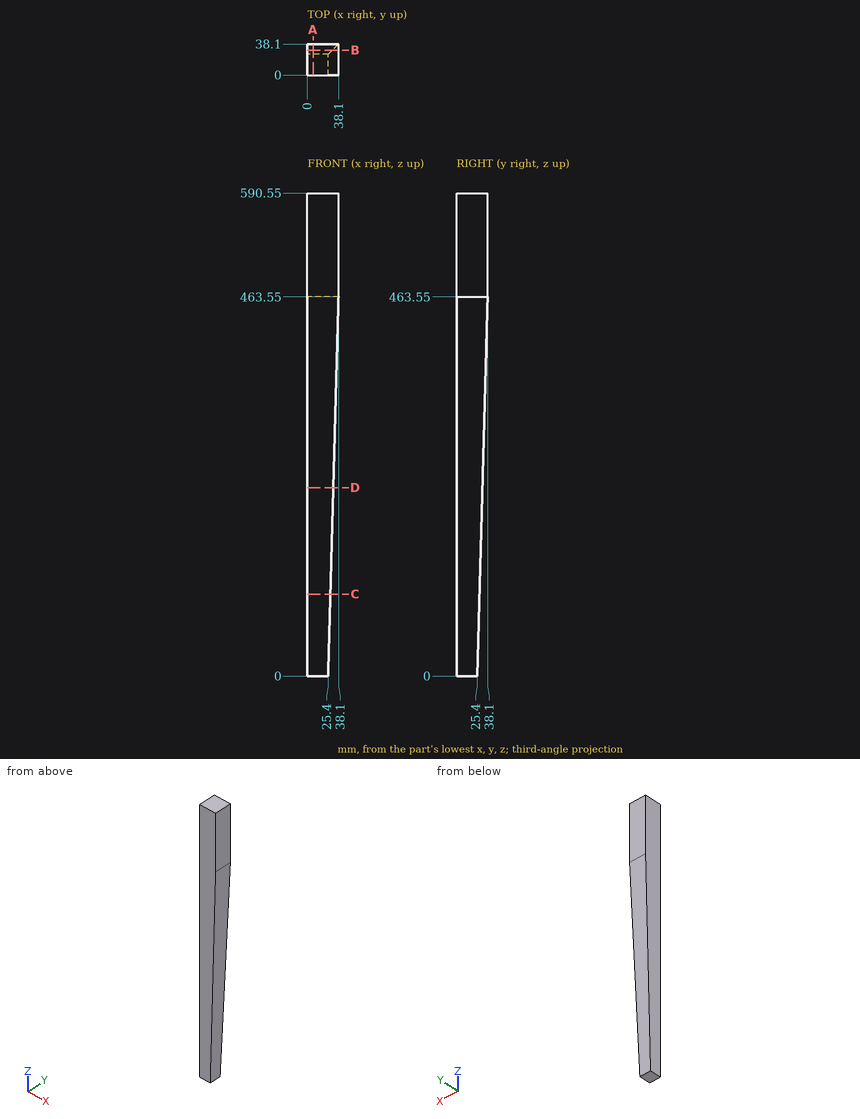
Source: three-view drawing plus pictorial views. Frame: mm from the lowest corner of the part. Round coordinates to 2 decimals unless told otherwise and drop trailing zeros. Order: outer loops, then holes, each group sorted by start corner. A loop starts at its lowest first (then second) coordinate and runs counter-clockwise, first axis right, second up. Notation, with made-up numbers: (7.5, 18.25) -> (33.5, 18.25) arc R24 ccw to (33.5, 57.25) -> close; hole circle Ø10 at (-16, 69). An arc over 180 degrees is marked (long way). Use one line per item in the form item = value. Start each with the question number.
1. Cut plane A-A (x = 7). Return the cut outline in (y, z), then the cut area to 3 significant figures.
2. Pin query (flat end, axial travel): pin 1 Ø4 at (x, z) = (23, 325.5) entering from +Y. Return the tip coordinate at first contact, or that it passes through.
3. Line query: probe 1 along X at (y, z) = (10, 186); probe 2 along X at (y, z) = (2, 153.5); probe 3 along Y at (x, z) = (21.5, 189). Output: solid intervals per line, ascending.
4. Cut plane B-B (y = 30.5). Return the cut outline in (x, z), then the cut area to 3 significant figures.
5. Cut plane C-C (z = 100). Return the cut outline in (x, y), then the cut area to 3 significant figures.
6. Cut plane D-D (z = 230.5). Return the cut outline in (x, y), then the cut area to 3 significant figures.
Solution:
q1.outline = (0, 0) -> (25.4, 0) -> (38.1, 463.55) -> (38.1, 590.55) -> (0, 590.55) -> close
q1.area = 19,600 mm^2
q2.pin_1 = 34.37
q3.probe_1 = 0 to 30.5
q3.probe_2 = 0 to 29.61
q3.probe_3 = 0 to 30.58
q4.outline = (0, 186.15) -> (30.5, 186.15) -> (38.1, 463.55) -> (38.1, 590.55) -> (0, 590.55) -> close
q4.area = 14,400 mm^2
q5.outline = (0, 0) -> (28.14, 0) -> (28.14, 28.14) -> (0, 28.14) -> close
q5.area = 792 mm^2
q6.outline = (0, 0) -> (31.72, 0) -> (31.72, 31.72) -> (0, 31.72) -> close
q6.area = 1,010 mm^2
